```python
from build123d import *

# Parameters (mm, degrees)
EXTRUDE_THIN1_DEPTH     = 40
CUT_EXTRUDE_THIN1_DEPTH = 10
CUT_EXTRUDE2_DEPTH      = 10


with BuildPart() as part:
    # Sketch1 → Extrude-Thin1 (new body)
    with BuildSketch(Plane.XY):
        with BuildLine():
            Line((0, 0), (-30, 0))
            Line((-30, 0), (-30, -30))
            ThreePointArc((-30, -30), (-24.142135624, -44.142135624), (-10, -50))
            Line((-10, -50), (20, -50))
            Line((20, -50), (20, -40))
            Line((20, -40), (-10, -40))
            ThreePointArc((-10, -40), (-17.071067812, -37.071067812), (-20, -30))
            Line((-20, -30), (-20, -10))
            Line((-20, -10), (0, -10))
            Line((0, -10), (0, 0))
        make_face()
    extrude(amount=EXTRUDE_THIN1_DEPTH)

    # Sketch3 → Cut-Extrude-Thin1 (cut)
    with BuildSketch(Plane(origin=(0, 0, 0), x_dir=(1, 0, 0), z_dir=(0, 1, 0))):
        with BuildLine():
            ThreePointArc((-10, -40), (-3.453740955, -37.676907189), (0, -31.650138477))
            Line((0, -31.650138477), (9.863069314, -33.299339409))
            ThreePointArc((9.863069314, -33.299339409), (2.955587404, -45.352876834), (-10.136930686, -49.999062455))
            Line((-10.136930686, -49.999062455), (-10, -40))
        make_face()
        with BuildLine():
            ThreePointArc((0, -10), (-2.928932188, -2.928932188), (-10, 0))
            Line((-10, 0), (-10, 10))
            ThreePointArc((-10, 10), (4.142135624, 4.142135624), (10, -10))
            Line((10, -10), (0, -10))
        make_face()
    extrude(amount=-CUT_EXTRUDE_THIN1_DEPTH, mode=Mode.SUBTRACT)

    # Sketch10 → Cut-Extrude2 (cut)
    with BuildSketch(Plane(origin=(0, -40, 0), x_dir=(1, 0, 0), z_dir=(0, 1, 0))):
        with BuildLine():
            ThreePointArc((0, 0), (14.142135624, -5.857864376), (20, -20))
            Line((20, -20), (20, 0))
            Line((20, 0), (0, 0))
        make_face()
        with BuildLine():
            ThreePointArc((20, -20), (14.142135624, -34.142135624), (0, -40))
            Line((0, -40), (20, -40))
            Line((20, -40), (20, -20))
        make_face()
        with BuildLine():
            ThreePointArc((0, -10), (-10, -20), (0, -30))
            Line((0, -30), (0, -10))
        make_face()
        with BuildLine():
            Line((0, -10), (0, -30))
            ThreePointArc((0, -30), (7.071067812, -27.071067812), (10, -20))
            ThreePointArc((10, -20), (7.071067812, -12.928932188), (0, -10))
        make_face()
    extrude(amount=-CUT_EXTRUDE2_DEPTH, mode=Mode.SUBTRACT)


solid = part.part
```
Here's how the part is built. I have some questions about the finished solid (model axes, mm). A direction names the side the tool comes from. Round coordinates to 2 decimals unless told otherwise and drop trailing zeros. Write each loop counter-clockwise with the first axis right and the second up, starting at its lowest first coordinate (ties: lowest second). Pieces come first, ordered by that corner, then holes.
Q1. Please list where these lines run through material, in increasing order: probe 1 along Y at (x, z) = (12.5, 18); probe 2 along X at (y, z) = (-13.5, 28); probe 3 along X at (y, z) = (-40.5, 26).
Q2. Which directions (+Z, -Z, +X, -X, +Y, -Y) give clear straight access to the entire face, cutting with the end or side of a thin tool? Please do faces 5 (the flat face through (-10, -10, 20)), 6 (the cylindrical face through (-2.85, -4.93, 3.01)), 7 (the cylindrical face through (-3.42, -4.93, 37.65)), 8 (the flat face through (-22, -25, 40)).
Q3. If we mould it in two halves opening along Y, with no side actions, what happens to faces 1 (the flat face through (12, -40, 20)), 2 (the flat face through (-22, -25, 0)), 3 (the cylindrical face through (-16.99, -37.15, 19.72)), 4 (the flat face through (11, -50, 20))? For each: +Y half, -Y half, draft (parallel to the pull), parting line (faces both ways), or undercut.
Q4. Will these pins go through, and if not, where does the flat tip stop? P1, Ø6, axis at x = 10.5, z = 9.5, coming from the +Y side; P2, Ø10, axis at y = -23, z = 23.5, coming from the +X side; P3, Ø6, axis at y = -7, z = 17.5, coming from the +X side.
Q5. If we section it at C-C on y = -8: Write out the boundary of the cut face in (x, z).
Q6. If we section it at D-D on x = -4: Write out the boundary of the cut face in (y, z), plus the area to 3 significant figures.
Q7. If we section it at B-B on z = 17: Write out the boundary of the cut face in (x, y), plus the area to 3 significant figures.
Q8. If we section it at A-A on x = 7: Write out the boundary of the cut face in (y, z) (3 decimals).
Answer below:
1. probe 1: y = -50 to -40
1. probe 2: x = -30 to -20
1. probe 3: x = -27.02 to -8, 8 to 19.08
2. face 5: +Z, -Z, +X
2. face 6: -Z, +X, +Y
2. face 7: +Z, +X, +Y
2. face 8: +Z, +X, -X, +Y, -Y
3. face 1: undercut
3. face 2: draft
3. face 3: undercut
3. face 4: -Y half
4. P1: stops at y = -40
4. P2: stops at x = -20
4. P3: stops at x = 0
5. outline: (-30, 0) - (-10, 0) arc R10 ccw to (0, 10) - (0, 31.65) arc R10 ccw to (-9.73, 40) - (-30, 40) - close
6. outline: (-50, 0) - (-40, 0) - (-40, 10.83) - (-50, 10.83) - close; (-50, 29.17) - (-40, 29.17) - (-40, 40) - (-50, 40) - close; (-10, 2) - (0, 2) - (0, 38.1) - (-10, 38.1) - close
6. area: 578 mm2
7. outline: (-30, -30) arc R20 ccw to (-10, -50) - (-9.54, -50) - (-9.54, -40) - (-10, -40) arc R10 cw to (-20, -30) - (-20, -10) - (0, -10) - (0, 0) - (-30, 0) - close; (9.54, -50) - (19.77, -50) - (19.77, -40) - (9.54, -40) - close
7. area: 843 mm2
8. outline: (-50, 1.265) - (-40, 1.265) - (-40, 12.859) - (-50, 12.859) - close; (-50, 27.141) - (-40, 27.141) - (-40, 38.735) - (-50, 38.735) - close
